Autodesk Inventor part; units mm, degrees
ref_plane "YZ Plane" through (0, 0, 0) normal (1, 0, 0) x (0, 1, 0)
ref_plane "XZ Plane" through (0, 0, 0) normal (0, 1, 0) x (-1, 0, 0)
ref_plane "XY Plane" through (0, 0, 0) normal (0, 0, 1) x (1, 0, 0)
sketch "Sketch2" plane through (0, 0, 0) normal (0, 0, 1) x (1, 0, 0)
  arc A0 (0, -52) -> (0, 52) centre (0, 0) ccw
  arc A1 (0, -50) -> (0, 50) centre (0, 0) ccw
  line L0 (0, 52) -> (0, 50)
  line L1 (0, -50) -> (0, -52)
  line L2 (0, -50) -> (2, -50)
  line L3 (2, -50) -> (2, -66)
  line L4 (2, -66) -> (0, -66)
  line L5 (0, -66) -> (0, -50)
  line L6 (0, 50) -> (2, 50)
  line L7 (2, 50) -> (2, 66)
  line L8 (2, 66) -> (0, 66)
  line L9 (0, 66) -> (0, 50)
  point P0 (0, 52)
  point P1 (2, 51.9615)
  point P2 (2, -51.9615)
  dimension "d0" = 104
  dimension "d1" = 100
  dimension "d2" = 2
  dimension "d5" = 2
  dimension "d6" = 16
  dimension "d7" = 2
  dimension "d8" = 16
extrude "Extrusion1" add sketch "Sketch2" along normal blind 80
fillet "Fillet1" radius 2 2 edges at (2, -51.9615, 40) (2, 51.9615, 40)
sketch "Sketch3" plane through (2, -66, 80) normal (1, 0, 0) x (0, 0, -1)
  line L0 (80, 16) -> (80, 0) construction
  line L1 (80, 0) -> (0, 0) construction
  line L2 (0, 16) -> (0, 0) construction
  line L3 (80, 16) -> (0, 16) construction
  line L4 (80, 132) -> (80, 116) construction
  line L5 (80, 116) -> (0, 116) construction
  line L6 (0, 132) -> (0, 116) construction
  line L7 (80, 132) -> (0, 132) construction
  point P0 (80, 66)
  point P1 (15, 6)
  point P2 (65, 6)
  point P3 (15, 126)
  point P4 (65, 126)
  dimension "d10" = 15
  dimension "d11" = 15
  dimension "d12" = 15
  dimension "d13" = 15
  dimension "d14" = 6
  dimension "d15" = 6
  dimension "d16" = 6
  dimension "d17" = 6
hole "Hole1" at (2, -60, 65) at (2, -60, 15) at (2, 60, 65) at (2, 60, 15) direction (-1, 0, 0) diameter 6.5 depth 2
sketch "Sketch4" plane through (0, 0, 0) normal (0, 1, 0) x (-1, 0, 0)
  line L0 (-3.8519, 80) -> (-3.8519, 0) construction
  line L1 (-3.8519, 80) -> (-3.8519, 80) construction
  line L2 (-3.8519, 0) -> (-3.8519, 80) construction
  line L3 (-3.8519, 0) -> (-3.8519, 0) construction
  line L4 (-52, 0) -> (-52, 80) construction
  line L5 (-50, 80) -> (-130, 80)
  line L6 (-130, 80) -> (-130, 65.4498)
  line L7 (-130, 65.4498) -> (-52, 0)
  line L8 (-52, 0) -> (-49.7983, 0)
  line L9 (-50, 80) -> (-50, 0) construction
  line L10 (-52, 0) -> (-50, 0)
  line L11 (-50, 0) -> (-50, 80)
  line L12 (-50, 80) -> (-50, 80)
  point P0 (0, 0)
  dimension "d25" = 80
  dimension "d26" = 130
extrude "Extrusion2" add sketch "Sketch4" along normal mid plane 4
sketch "Sketch5" plane through (0, -2, 0) normal (0, -1, 0) x (1, 0, 0)
  line L0 (130, 80) -> (51.9615, 80) construction
  line L1 (130, 65.4498) -> (130, 80) construction
  point P0 (0, 0)
  point P1 (115, 70)
  point P2 (52, 80)
  dimension "d29" = 10
  dimension "d30" = 15
hole "Hole2" at (115, -2, 70) direction (0, 1, 0) diameter 9 depth 4
fillet "Fillet2" radius 2 2 edges at (130, 0, 80) (130, 0, 65.4498)
fillet "Fillet3" radius 2 2 edges at (51.9615, -2, 40) (51.9615, 2, 40)
properties part number "P049_SupportTube"
Geometry check sheet. Reference: the model listing, model coordinates, mm. A direction names the side the tool comes from. Give positions to 0.01 mm unless a question says otherwise; leave off trailing zeros. Loops run counter-clockwise (first coordinate to the right, second up) from the corner with the lowest first, then second, coordinate; pieces in that order, holes last. Notation, with made-up numbers: (36.5, 80.25) -> (67.5, 80.25) arc R17 cw to (67.5, 112.25) -> close; hole circle Ø4 at (39.25, 39.25). An arc over 180 degrees is marked (long way). Answer in a Markdown table with one row per item. Add a question column.
1) Cross-section at A-A on z = 70. Record the boundary of the cut face in (x, y), and give its area (3 significant figures).
2) Cross-section at D-D on y = -60. Record the boundary of the cut face in (x, z).
3) Material ranges on probe 1 along Y at (x, z) = (0.9, 65); probe 2 along Z at (x, y) = (0.9, 60); probe 3 along Y at (x, z) = (76.5, 74), recorded low to high. Write a range as from..to.
4) Set-up check for faces 5 (the face through (84, 2, 50)), 6 (the face through (2, -60, 39)), 7 (the face through (0, -58, 39)): record each of +Z, -Z, +X, -X, +Y, -Y from which the full face is reachable in a straight line by a thin tool's end or side.
5) Draft check along Y on faces 1 (the face through (37.134, -36.402, 39.44)), 2 (the face through (36.402, 37.134, 39.44)), 3 (the face through (49.988, 1.099, 39.44)), 4 (the face through (130, 0, 72)). Enter one of: pulls with the +Y half, pulls with the -Y half, needs draft (parallel to the pull), parting line crosses it, or undercut.
6) Cross-section at B-B on y = 0. Record the boundary of the cut face in (x, z).
7) Gauge pin test, flat ends, axial feed: P1, Ø6, axis at x = 107, y = 7, coming from the -Z side; P2, Ø6, axis at y = 58.5, z = 23, coming from the +X side; P3, Ø4, axis at y = 37.5, z = 57, coming from the +X side; P4, Ø1, axis at y = -32.5, z = 69.5, coming from the +X side. Record the tip position at first contact, or that the pin passes through.
8) Cross-section at C-C on x = 48. Record the boundary of the cut face in (y, z).
Outcome:
| question | item | result |
|---|---|---|
| 1 | outline | (0, -66) -> (2, -66) -> (2, -53.85) arc R2 cw to (3.85, -51.86) arc R52 ccw to (51.86, -3.85) arc R2 cw to (53.85, -2) -> (110.5, -2) -> (110.5, 2) -> (53.85, 2) arc R2 cw to (51.86, 3.85) arc R52 ccw to (3.85, 51.86) arc R2 cw to (2, 53.85) -> (2, 66) -> (0, 66) -> (0, 50) arc R50 cw to (0, -50) -> close; (119.5, -2) -> (130, -2) -> (130, 2) -> (119.5, 2) -> close |
| 1 | area | 656 mm^2 |
| 2 | outline | (0, 0) -> (2, 0) -> (2, 11.75) -> (0, 11.75) -> close; (0, 18.25) -> (2, 18.25) -> (2, 61.75) -> (0, 61.75) -> close; (0, 68.25) -> (2, 68.25) -> (2, 80) -> (0, 80) -> close |
| 3 | probe 1 | y = -66..-63.25, -56.75..-49.99, 49.99..56.75, 63.25..66 |
| 3 | probe 2 | z = 0..11.75, 18.25..61.75, 68.25..80 |
| 3 | probe 3 | y = -2..2 |
| 4 | face 5 | +Z, -Z, +X, +Y |
| 4 | face 6 | +Z, -Z, +X, -Y |
| 4 | face 7 | +Z, -Z, -X, +Y, -Y |
| 5 | face 1 | pulls with the -Y half |
| 5 | face 2 | pulls with the +Y half |
| 5 | face 3 | undercut |
| 5 | face 4 | needs draft |
| 6 | outline | (50, 0) -> (52, 0) -> (129.29, 64.85) arc R2 ccw to (130, 66.38) -> (130, 78) arc R2 ccw to (128, 80) -> (50, 80) -> close; hole circle Ø9 at (115, 70) |
| 7 | P1 | passes through |
| 7 | P2 | stops at x = 2 |
| 7 | P3 | stops at x = 38 |
| 7 | P4 | stops at x = 40.99 |
| 8 | outline | (-20, 0) -> (-14, 0) -> (-14, 80) -> (-20, 80) -> close; (14, 0) -> (20, 0) -> (20, 80) -> (14, 80) -> close |
